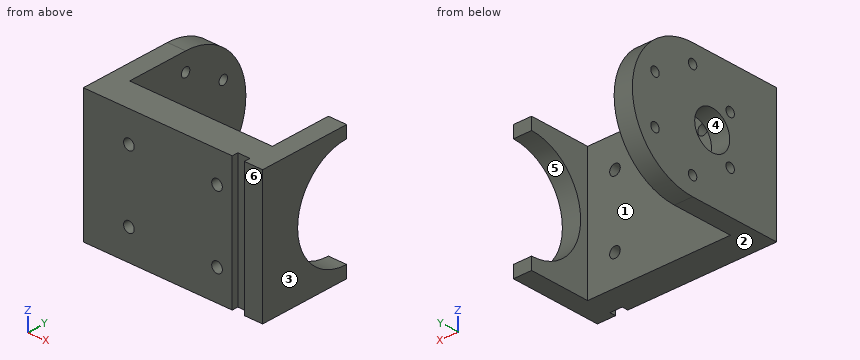
from build123d import *

# Parameters (mm, degrees)
SKETCH1_W           = 59
SKETCH1_H           = 43
SKETCH1_R           = 1.75
BOSS_EXTRUDE1_DEPTH = 10
SKETCH2_W           = 4
SKETCH2_H           = 43
CUT_EXTRUDE1_DEPTH  = 2
BOSS_EXTRUDE2_DEPTH = 6
SKETCH5_R           = 6.25
SKETCH5_R_2         = 1.5
BOSS_EXTRUDE3_DEPTH = 6


with BuildPart() as part:
    # Sketch1 → Boss-Extrude1 (new body)
    with BuildSketch(Plane(origin=(0, 0, 0), x_dir=(1, 0, 0), z_dir=(0, 1, 0))):
        with Locations((29.5, 21.5)):
            Rectangle(SKETCH1_W, SKETCH1_H)
        with Locations(Location((15, 33, 0), (0, 0, 270))):
            Circle(SKETCH1_R, mode=Mode.SUBTRACT)
        with Locations(Location((15, 10, 0), (0, 0, 90))):
            Circle(SKETCH1_R, mode=Mode.SUBTRACT)
        with Locations(Location((44, 33, 0), (0, 0, 90))):
            Circle(SKETCH1_R, mode=Mode.SUBTRACT)
        with Locations(Location((44, 10, 0), (0, 0, 270))):
            Circle(SKETCH1_R, mode=Mode.SUBTRACT)
    extrude(amount=BOSS_EXTRUDE1_DEPTH)

    # Sketch2 → Cut-Extrude1 (cut)
    with BuildSketch(Plane.XZ):
        with Locations((51, -21.5)):
            Rectangle(SKETCH2_W, SKETCH2_H)
    extrude(amount=-CUT_EXTRUDE1_DEPTH, mode=Mode.SUBTRACT)

    # Sketch3 → Boss-Extrude2 (add)
    with BuildSketch(Plane(origin=(59, 0, 0), x_dir=(0, 0, -1), z_dir=(1, 0, 0))):
        with BuildLine():
            Line((0, 10), (43, 10))
            Line((43, 10), (43, 30))
            Line((43, 30), (39, 30))
            ThreePointArc((39, 30), (21.5, 12.5), (4, 30))
            Line((4, 30), (0, 30))
            Line((0, 30), (0, 10))
        make_face()
    extrude(amount=-BOSS_EXTRUDE2_DEPTH)

    # Sketch5 → Boss-Extrude3 (add)
    with BuildSketch(Plane.ZY):
        with BuildLine():
            Line((-43, 10), (0, 10))
            Line((0, 10), (0, 30))
            ThreePointArc((0, 30), (-21.5, 51.5), (-43, 30))
            Line((-43, 30), (-43, 10))
        make_face()
        with Locations((-21.5, 23)):
            Circle(SKETCH5_R, mode=Mode.SUBTRACT)
        with Locations((-6, 30)):
            Circle(SKETCH5_R_2, mode=Mode.SUBTRACT)
        with Locations((-13.75, 16.576606241)):
            Circle(SKETCH5_R_2, mode=Mode.SUBTRACT)
        with Locations((-29.25, 16.576606241)):
            Circle(SKETCH5_R_2, mode=Mode.SUBTRACT)
        with Locations((-37, 30)):
            Circle(SKETCH5_R_2, mode=Mode.SUBTRACT)
        with Locations((-29.25, 43.423393759)):
            Circle(SKETCH5_R_2, mode=Mode.SUBTRACT)
        with Locations((-13.75, 43.423393759)):
            Circle(SKETCH5_R_2, mode=Mode.SUBTRACT)
    extrude(amount=-BOSS_EXTRUDE3_DEPTH)


solid = part.part
Geometry: final body of the model. Coordinates: model frame, mm. Face numbers are marked on the shaded views. A direction names the side the tool comes from. Round coordinates to 2 decimals unless told otherwise and drop trailing zeros. Loops run counter-clockwise (first coordinate to the right, second up) from the corner with the lowest first, then second, coordinate; pieces in that order, holes last. Notation, with made-up numbers: M 64,7.5 L 102,7.5 A14 ccw 102,12.5 Z; hole C 17,-27 d8. An arc over 180 degrees is marked long. Put each result on its own line as item: value. Start each with the question number.
(1) Section query D-D (y = 19). Return loops of the section in (x, z), then the cut area to 3 significant figures.
(2) Section query A-A (z = -21.5). Return loops of the section in (x, y), then the cut area to 3 significant figures.
(3) Section query C-C (x = 15). Return loops of the section in (y, z).
(4) Contact query for flat-ended pins moving along their axis: pin 1 Ø3 at (x, z) = (44, -10) entering from -Y; pin 2 Ø2 at (x, z) = (55, -2) entering from +Y; pin 3 Ø1 at (x, z) = (42, -21) entering from +Y; pin 4 Ø3.5 at (y, z) = (30, -6) entering from +X. Output: stop coordinate, or through.
(5) Material intervals for line 1 along X through (y, z) = (22, -2); line 2 along X through (y, z) = (6, -10); line 3 along Y through (x, z) = (24.5, -36.5), sorted ascending. Write a range as [from, to].
(6) Set-up query: the marked faces 1 and 2. Return all of +Z, -Z, +X, -X, +Y, -Y with unobstructed straight access to the full face (end or side cutting, diameter ignored); none if empty.
(7) Draft query along Y for the marked faces 3, 4, 5 and 6. Return one class per face: +Y half, -Y half, draft (parallel to the pull), parting line (faces both ways), or undercut.
(8) Section query B-B (y = 5.5). Return loops of the section in (x, z), then the cut area to 3 significant figures.
Findings below:
1. outline: M 0,-43 L 6,-43 L 6,-26.3 L 0,-26.3 Z; M 0,-16.7 L 6,-16.7 L 6,0 L 0,0 Z; M 53,-43 L 59,-43 L 59,-35.11 L 53,-35.11 Z; M 53,-7.89 L 59,-7.89 L 59,0 L 53,0 Z
1. area: 295 mm2
2. outline: M 0,0 L 49,0 L 49,2 L 53,2 L 53,0 L 59,0 L 59,12.5 L 53,12.5 L 53,10 L 6,10 L 6,16.75 L 0,16.75 Z; M 0,29.25 L 6,29.25 L 6,51.5 L 0,51.5 Z
2. area: 771 mm2
3. outline: M 0,-43 L 10,-43 L 10,-34.75 L 0,-34.75 Z; M 0,-31.25 L 10,-31.25 L 10,-11.75 L 0,-11.75 Z; M 0,-8.25 L 10,-8.25 L 10,0 L 0,0 Z
4. pin 1: passes through
4. pin 2: stops at y = 30
4. pin 3: stops at y = 10
4. pin 4: stops at x = 6
5. line 1: x = [0, 6], [53, 59]
5. line 2: x = [0, 13.25], [16.75, 42.25], [45.75, 59]
5. line 3: y = [0, 10]
6. face 1: +Z, -Z, +Y
6. face 2: -Z, +X, -X, +Y, -Y
7. face 3: draft
7. face 4: undercut
7. face 5: +Y half
7. face 6: -Y half
8. outline: M 0,-43 L 59,-43 L 59,0 L 0,0 Z; hole C 15,-33 d3.5; hole C 15,-10 d3.5; hole C 44,-33 d3.5; hole C 44,-10 d3.5
8. area: 2,500 mm2
